Geometry: final body of the model. Coordinates: model frame, mm. Face numbers are marked on the shaded views. A direction names the side the tool comes from. Give positions to 0.01 mm unless a question says otherwise; leave off trailing zeros. Loops run counter-clockwise (first coordinate to the right, second up) from the corner with the lowest first, then second, coordinate; pieces in that order, holes last. Notation, with made-up numbers: (-22, 68) - (-13, 68) arc R33 cw to (-13, 97) - close; hole circle Ø8 at (-37, -3.75). An arc over 180 degrees is marked (long way). Answer in a Markdown table with one row per item.
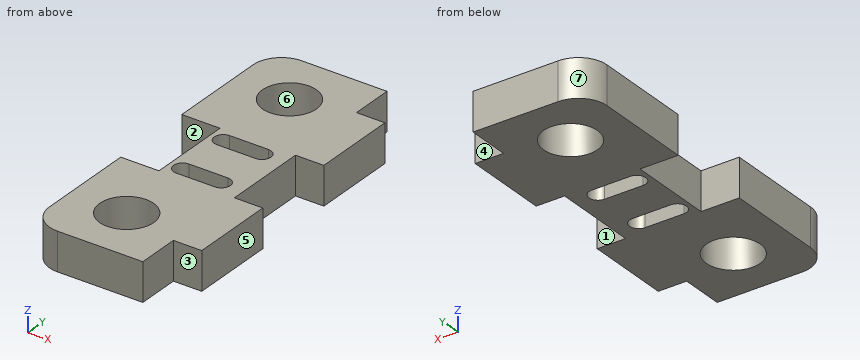
Autodesk Inventor part; units mm, degrees
ref_plane "YZ Plane" through (0, 0, 0) normal (1, 0, 0) x (0, 1, 0)
ref_plane "XZ Plane" through (0, 0, 0) normal (0, 1, 0) x (-1, 0, 0)
ref_plane "XY Plane" through (0, 0, 0) normal (0, 0, 1) x (1, 0, 0)
sketch "Sketch1" plane through (0, 0, 0) normal (0, 0, 1) x (1, 0, 0)
  line L0 (0, 0) -> (0, 60)
  line L1 (0, 60) -> (20, 60)
  line L2 (20, 60) -> (20, 52.5)
  line L3 (20, 52.5) -> (25, 52.5)
  line L4 (25, 52.5) -> (25, 37.5)
  line L5 (25, 37.5) -> (20, 37.5)
  line L6 (20, 37.5) -> (20, 22.5)
  line L7 (20, 22.5) -> (25, 22.5)
  line L8 (25, 22.5) -> (25, 7.5)
  line L9 (25, 7.5) -> (20, 7.5)
  line L10 (20, 7.5) -> (20, 0)
  line L11 (20, 0) -> (0, 0)
  circle A0 centre (10, 10) radius 4.75
  circle A1 centre (10, 50) radius 4.75
  circle A2 centre (5, 41.25) radius 1.59
  circle A3 centre (12.5, 30) radius 1.59
  line L12 (7.5, 36.5875) -> (17.5, 36.5875)
  line L13 (17.5, 36.5875) -> (17.5, 33.4125)
  line L14 (17.5, 33.4125) -> (7.5, 33.4125)
  line L15 (7.5, 33.4125) -> (7.5, 36.5875)
  line L16 (7.5, 26.5875) -> (17.5, 26.5875)
  line L17 (17.5, 26.5875) -> (17.5, 23.4125)
  line L18 (17.5, 23.4125) -> (7.5, 23.4125)
  line L19 (7.5, 23.4125) -> (7.5, 26.5875)
  line L20 (9.0875, 35) -> (15.9125, 35) construction
  line L21 (9.0875, 33.4125) -> (15.9125, 33.4125)
  line L22 (15.9125, 36.5875) -> (9.0875, 36.5875)
  arc A4 (9.0875, 36.5875) -> (9.0875, 33.4125) centre (9.0875, 35) ccw
  arc A5 (15.9125, 33.4125) -> (15.9125, 36.5875) centre (15.9125, 35) ccw
  line L23 (9.0875, 25) -> (15.9125, 25) construction
  line L24 (9.0875, 23.4125) -> (15.9125, 23.4125)
  line L25 (15.9125, 26.5875) -> (9.0875, 26.5875)
  arc A6 (9.0875, 26.5875) -> (9.0875, 23.4125) centre (9.0875, 25) ccw
  arc A7 (15.9125, 23.4125) -> (15.9125, 26.5875) centre (15.9125, 25) ccw
  point P0 (12.5, 35)
  point P1 (12.5, 25)
  point P2 (20, 30)
  dimension "d0" = 15
  dimension "d1" = 60
  dimension "d2" = 20
  dimension "d3" = 5
  dimension "d6" = 9.5
  dimension "d7" = 40
  dimension "d8" = 10
  dimension "d9" = 10
  dimension "d11" = 10
  dimension "d12" = 10
  dimension "d25" = 3.18
  dimension "d26" = 15
  dimension "d29" = 2.5
  dimension "d30" = 3.175
  dimension "d33" = 10
  dimension "d34" = 10
  dimension "d35" = 5
  dimension "d36" = 7.5
  dimension "d37" = 11.25
extrude "Extrusion1" add sketch "Sketch1" along normal blind 6.731 contours L0 L1 L2 L3 L4 L5 L6 L7 L8 L9 L10 L11 | A2 | A3 | L12 A4 L15 | L12 A5 L14 A4 | A4 L14 L15 | L12 L13 A5 | L13 L14 A5 | L16 A6 L19 | L16 A7 L18 A6 | A6 L18 L19 | L16 L17 A7 | L17 L18 A7
sketch "Sketch2" plane through (0, 0, 0) normal (0, 0, -1) x (-1, 0, 0)
  line L0 (0, 0) -> (-20, 0)
  line L1 (0, 60) -> (0, 0)
  line L2 (-20, 22.5) -> (-20, 37.5)
  line L3 (0, 22.5) -> (-6.731, 22.5)
  line L4 (-6.731, 22.5) -> (-6.731, 37.5)
  line L5 (-6.731, 37.5) -> (0, 37.5)
  line L6 (0, 37.5) -> (0, 22.5)
  line L7 (-9.0875, 25) -> (-15.9125, 25) construction
  line L8 (-9.0875, 26.5875) -> (-15.9125, 26.5875)
  line L9 (-15.9125, 23.4125) -> (-9.0875, 23.4125)
  arc A0 (-9.0875, 23.4125) -> (-9.0875, 26.5875) centre (-9.0875, 25) ccw
  arc A1 (-15.9125, 26.5875) -> (-15.9125, 23.4125) centre (-15.9125, 25) ccw
  line L10 (-9.0875, 35) -> (-15.9125, 35) construction
  line L11 (-9.0875, 36.5875) -> (-15.9125, 36.5875)
  line L12 (-15.9125, 33.4125) -> (-9.0875, 33.4125)
  arc A2 (-9.0875, 33.4125) -> (-9.0875, 36.5875) centre (-9.0875, 35) ccw
  arc A3 (-15.9125, 36.5875) -> (-15.9125, 33.4125) centre (-15.9125, 35) ccw
  point P0 (0, 30)
  point P1 (0, 30)
  point P2 (-12.5, 25)
  point P3 (-12.5, 35)
  dimension "d38" = 6.731
  dimension "d39" = 15
  dimension "d40" = 10
  dimension "d41" = 3.175
  dimension "d42" = 6.825
  dimension "d43" = 2.5
  dimension "d44" = 5
extrude "Extrusion2" cut sketch "Sketch2" against normal up to next
fillet "Fillet1" radius 5 2 edges at (0, 60, 3.3655) (0, 0, 3.3655)
equation "\"d6\" = MAGDIA"
equation "\"d8\" = d9"
equation "\"d11\" = d12"
equation "\"d4\" = THICKB"
equation "\"d38\" = THICKB"
equation "\"THICKA\" = 3.175"
equation "\"THICKB\" = 6.731"
equation "\"THICKC\" = 12.7"
equation "\"MAGDIA\" = 9.5"
equation "\"BALLDIA\" = 12"
equation "\"THICKPLY\" = 5"
properties part number "Carriage_Joint_Frame"
Q1. Cut plane C-C (x = 10). Output: boundary loops of the cut face in (y, z), and give its area (3 significant figures).
Check values:
| item | result |
|---|---|
| outline | (0, 0) - (5.25, 0) - (5.25, 6.73) - (0, 6.73) - close; (14.75, 0) - (23.41, 0) - (23.41, 6.73) - (14.75, 6.73) - close; (26.59, 0) - (33.41, 0) - (33.41, 6.73) - (26.59, 6.73) - close; (36.59, 0) - (45.25, 0) - (45.25, 6.73) - (36.59, 6.73) - close; (54.75, 0) - (60, 0) - (60, 6.73) - (54.75, 6.73) - close |
| area | 233 mm² |
Q2. Cut plane A-A (x = 2). Output: boundary loops of the cut face in (y, z).
Check values:
| item | result |
|---|---|
| outline | (1, 0) - (22.5, 0) - (22.5, 6.73) - (1, 6.73) - close; (37.5, 0) - (59, 0) - (59, 6.73) - (37.5, 6.73) - close |
Q3. Material intervals for line 1 along Y through (x, z) = (10, 2.5); line 2 along X through (y, z) = (35, 1); line 3 along Y through (x, z) = (20.25, 4.5), sorted ascending.
Check values:
| item | result |
|---|---|
| line 1 | 0 to 5.25, 14.75 to 23.41, 26.59 to 33.41, 36.59 to 45.25, 54.75 to 60 |
| line 2 | 6.73 to 7.5, 17.5 to 20 |
| line 3 | 7.5 to 22.5, 37.5 to 52.5 |
Q4. Draft query along Y for the marked faces 5, 6 and 7. Return one class per face: pulls with the +Y half, pulls with the -Y half, needs draft (parallel to the pull), parting line crosses it, or undercut.
Check values:
| item | result |
|---|---|
| face 5 | needs draft |
| face 6 | undercut |
| face 7 | pulls with the +Y half |
Q5. Cut plane B-B (y = 10). Output: boundary loops of the cut face in (x, z).
Check values:
| item | result |
|---|---|
| outline | (0, 0) - (5.25, 0) - (5.25, 6.73) - (0, 6.73) - close; (14.75, 0) - (25, 0) - (25, 6.73) - (14.75, 6.73) - close |
Q6. First-contact query: pin 1 (1.5 mm diameter, centred on x = 23, z = 2, fed in from -Y); pin 2 (2 mm diameter, centred on y = 27, z = 3.5, fed in from +X); pin 3 (3 mm diameter, centred on x = 22.5, z = 3, fed in from +Y). Flat tips, straight axial feed; report the tip coordinate or a pass-through.
Check values:
| item | result |
|---|---|
| pin 1 | y = 7.5 |
| pin 2 | x = 20 |
| pin 3 | y = 52.5 |
Q7. Cut plane D-D (z = 4.5). Give the number of separate pieces and of enclosed holes in the cut face, and give its area (3 significant figures).
Check values:
| item | result |
|---|---|
| separate pieces | 1 |
| enclosed holes | 4 |
| area | 1,040 mm² |
Q8. Reachability of the marked faces 1, 2, 3 and 4 from +Z, -Z, +X, -X, +Y, -Y: full face, straight path, thin tool, end or side. Return the list, or none.
Check values:
| item | result |
|---|---|
| face 1 | +Z, -Z, +X |
| face 2 | +Z, -Z, -X |
| face 3 | +Z, -Z, +X, -Y |
| face 4 | +Z, -Z, +X, +Y |
